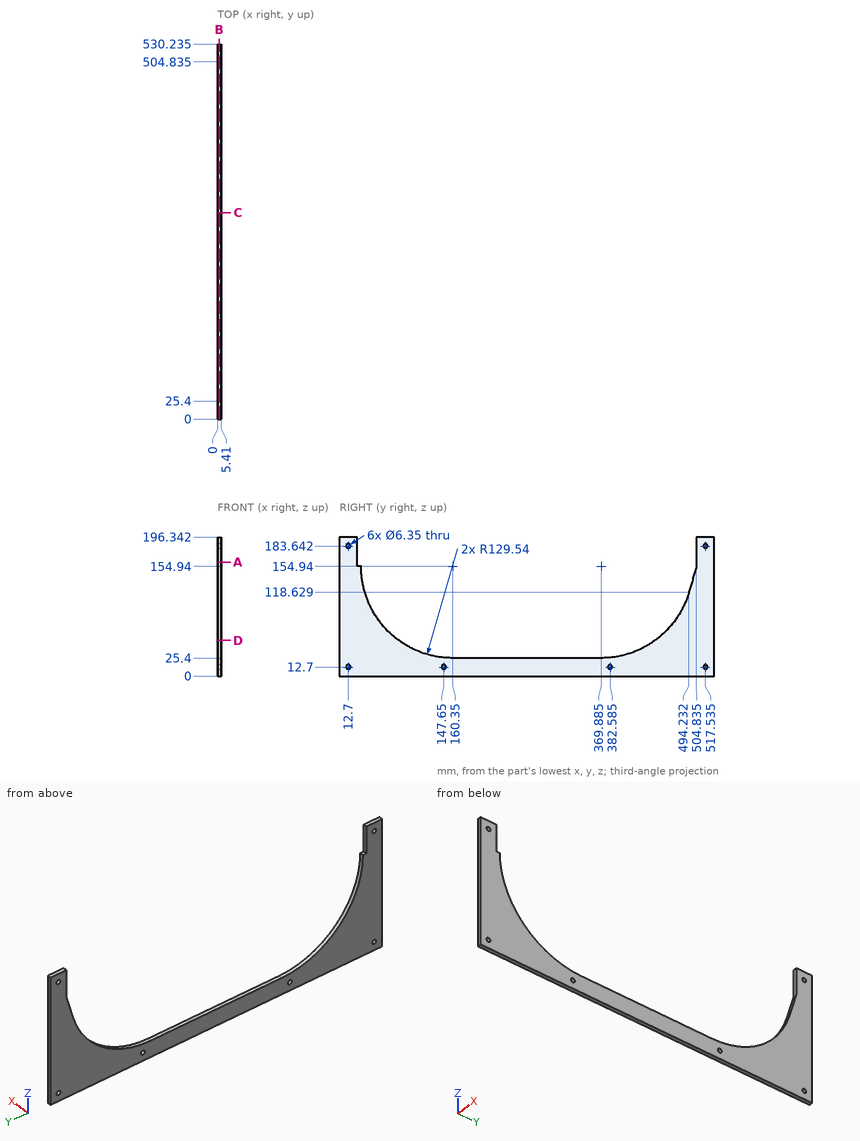
The drawing under review shows one solid part. Ordinate dimensions are in mm from its lowest x, y, z. Give positions to 0.01 mm unless a question says otherwise; leave off trailing zeros. Write each loop counter-clockwise with the first axis right and the second up, starting at its lowest first coordinate (ties: lowest second). Pieces come first, ordered by that corner, then holes.
1. Add section D-D, the plane z = 50.5. Write out the cut boundary in (x, y) (1 decimal), plus the area to 3 significant figures.
2. For P1, Ø4, axis at y = 147.65, z = 12.7, coming from the +X side; P2, Ø3, axis at x = 5, y = 451.5, coming from the +Z side, all flat-tipped, find the tip position at first contact; note any pin that passes through.
3. Add section B-B, the plane x = 2.3. Count the separate pieces of the cut face and the enclosed holes in it, plus the area to 3 significant figures.
4. Wall thickness on L1, parallel to Y at x = 4.85, z = 160 (1 decimal); L2, parallel to Z at x = 5.15, y = 331.5; L3, parallel to Y at x = 2.45, z = 98.5 (1 decimal): over which ranges is each line inside the solid? List them lowest first.
5. Add section C-C, the plane y = 292. Write out the cut boundary in (x, z), plus the area to 3 significant figures.
6. Add section A-A, the plane z = 161. Write out the cut boundary in (x, y) (1 decimal).
Worked answers:
1. outline: (0, 0) - (5.4, 0) - (5.4, 83.7) - (0, 83.7) - close; (0, 446.5) - (5.4, 446.5) - (5.4, 530.2) - (0, 530.2) - close
1. area: 906 mm2
2. P1: passes through
2. P2: stops at z = 55.58
3. separate pieces: 1
3. enclosed holes: 6
3. area: 30,500 mm2
4. L1: y = 0 to 25.4, 504.8 to 530.2
4. L2: z = 0 to 25.4
4. L3: y = 0 to 43.8, 486.5 to 530.2
5. outline: (0, 0) - (5.41, 0) - (5.41, 25.4) - (0, 25.4) - close
5. area: 137 mm2
6. outline: (0, 0) - (5.4, 0) - (5.4, 25.4) - (0, 25.4) - close; (0, 504.8) - (5.4, 504.8) - (5.4, 530.2) - (0, 530.2) - close
